Verification items for this drawing (mm, ordinates from the low corner). A direction names the side the tool comes from. Round coordinates to 2 decimals unless told otherwise and drop trailing zeros. Order: outer loops, then holes, each group sorted by start corner. A loop starts at its lowest first (then second) coordinate and runs counter-clockwise, first axis right, second up. Notation, with made-up numbers: (81, 67) - (93, 67) arc R27 ccw to (93, 96) - close; hole circle Ø2 at (13.5, 55.5). An arc over 180 degrees is marked (long way). One line per question, with ' | ' between items. Start each with the question number.
Q1. Sectioned sample at B-B, the plane z = 10.25. Enter the section's corners in (x, y).
Q2. Gauge pin test, flat ends, axial feed: P1, Ø3, axis at y = 5.5, z = 7, coming from the +X side; P2, Ø1, axis at y = 4, z = 4, coming from the -X side; P3, Ø8, axis at x = 8, z = 6.5, coming from the -Y side. Record the tip position at first contact, or that the pin passes through.
Q3. Mould release check, pull along Y, two halves, no side actions. Record for the marked faces 1, 2 and 3: +Y half, -Y half, draft (parallel to the pull), parting line (faces both ways), or undercut.
Q4. Material ranges on line 1 along Y through (x, z) = (7, 13.25); line 2 along Z through (x, y) = (7, 12.5); line 3 along X through (y, z) = (8.75, 4.25), recorded low to high.
Q5. Tool access check on the marked faces 4 and 5. Record the directions out of +Z, -Z, +X, -X, +Y, -Y that give a thin tool (end or side, any length) a straight path to the whole face; none if there is none.
Q6. Sectioned sample at A-A, the plane x = 7. Enter the section's corners in (y, z), then the cut area to 3 significant figures.
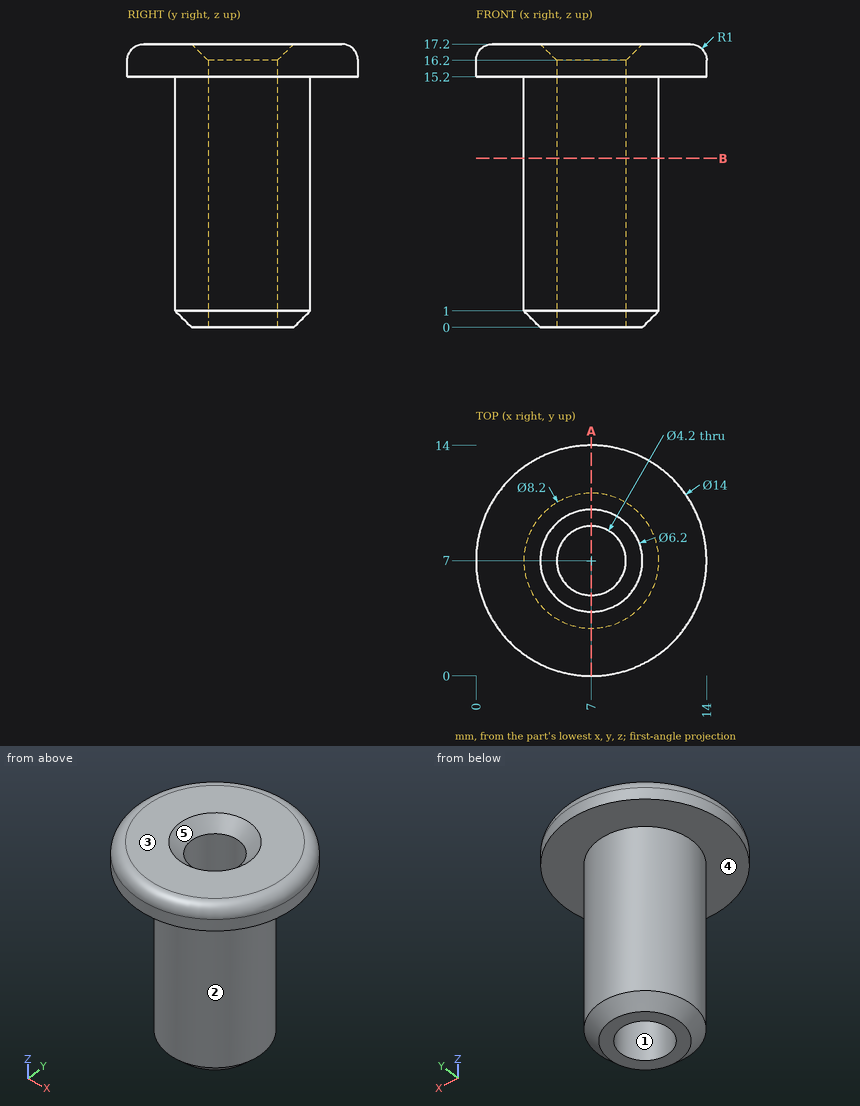
Determined:
1) outline: circle Ø8.2 at (7, 7); hole circle Ø4.2 at (7, 7)
2) P1: stops at x = 11.1 | P2: stops at x = 3.75 | P3: stops at y = 2.9
3) face 1: undercut | face 2: parting line | face 3: draft
4) line 1: y = 2.9 to 4.9, 9.1 to 11.1 | line 2: z = 15.2 to 17.2 | line 3: x = 3.29 to 5.84, 8.16 to 10.71
5) face 4: -Z | face 5: +Z
6) outline: (0, 15.2) - (2.9, 15.2) - (2.9, 1) - (3.9, 0) - (4.9, 0) - (4.9, 16.2) - (3.9, 17.2) - (1, 17.2) arc R1 ccw to (0, 16.2) - close; (9.1, 0) - (10.1, 0) - (11.1, 1) - (11.1, 15.2) - (14, 15.2) - (14, 16.2) arc R1 ccw to (13, 17.2) - (10.1, 17.2) - (9.1, 16.2) - close | area: 78.0 mm2
